Build history of the part. All positions in model axes, mm. Round coordinates to 2 decimals unless told otherwise and drop trailing zeros. Order: outer loops, then holes, each group sorted by start corner. A loop starts at its lowest first (then second) coordinate and runs counter-clockwise, first axis right, second up. Notation, with made-up numbers: (73.5, 15) - (128.5, 15) arc R29 cw to (128.5, 39) - close; hole circle Ø4 at (12.25, -18). An arc over 180 degrees is marked (long way). One line per question, with ' | ' between items. Start each with the question number.
from build123d import *

# Parameters (mm, degrees)
EXTRUDE_1_DEPTH   = 2
HOLE_WIZARD_M81_D = 9
CHAMFER_1_SIZE    = 2


with BuildPart() as part:
    # Эскиз1 → Бобышка-Вытянуть1 (new body)
    with BuildSketch(Plane(origin=(0, 0, 0), x_dir=(1, 0, 0), z_dir=(0, 0, -1))):
        Polygon((-75, 150), (75, 150), (75, 100), (25, 100), (25, 0), (-25, 0), (-25, 100), (-75, 100), align=None)
    extrude(amount=EXTRUDE_1_DEPTH)

    # Отверстие с зазором M81 (through all)
    with Locations(Plane(origin=(0, 0, -2), x_dir=(1, 0, 0), z_dir=(0, 0, -1))):
        with Locations((0, 25), (0, 125), (-50, 125), (50, 125), (0, 75)):
            Hole(HOLE_WIZARD_M81_D / 2)

    # Фаска1
    chamfer_1_edges = [part.edges().sort_by_distance(p)[0] for p in [
        (-75, -100, -1),
        (-75, -150, -1),
        (75, -150, -1),
        (75, -100, -1),
        (25, 0, -1),
        (-25, 0, -1),
    ]]
    chamfer(chamfer_1_edges, length=CHAMFER_1_SIZE)


solid = part.part
Item 1: Slice it at B-B (z = -0.4). Write the cut outline in (x, y), plus the area to 3 significant figures.
Item 2: Slice it at A-A (x = -50). Write the cut outline in (y, z).
Item 3: Wall check: line 1 along X through (y, z) = (-125, -0.55); line 2 along Y through (x, z) = (0, -1.1); line 3 along Y through (x, z) = (50, -1). Give the ranges that are in metal, low to high. Write a range as [from, to].
Item 4: Pin check, flat tips, straight feed: pin 1 (7 mm diameter, centred on x = 0, y = -125, fed in from -Z); pin 2 (1 mm diameter, centred on x = 39, z = -1, fed in from +Y); pin 3 (1 mm diameter, centred on y = -56.5, z = -1, fed in from -X); pin 4 (0.6 mm diameter, centred on y = -46.5, z = -1, fed in from +X). Stop position of each tip, or through.
Item 5: Slice it at D-D (x = 0). Write the cut outline in (y, z).
Item 6: Slice it at C-C (y = -25). Write the cut outline in (x, z), plus the area to 3 significant figures.
A:
1) outline: (-75, -148) - (-73, -150) - (73, -150) - (75, -148) - (75, -102) - (73, -100) - (25, -100) - (25, -2) - (23, 0) - (-23, 0) - (-25, -2) - (-25, -100) - (-73, -100) - (-75, -102) - close; hole circle Ø9 at (-50, -125); hole circle Ø9 at (0, -125); hole circle Ø9 at (0, -75); hole circle Ø9 at (0, -25); hole circle Ø9 at (50, -125) | area: 12,200 mm^2
2) outline: (-150, -2) - (-129.5, -2) - (-129.5, 0) - (-150, 0) - close; (-120.5, -2) - (-100, -2) - (-100, 0) - (-120.5, 0) - close
3) line 1: [-75, -54.5], [-45.5, -4.5], [4.5, 45.5], [54.5, 75] | line 2: [-150, -129.5], [-120.5, -79.5], [-70.5, -29.5], [-20.5, 0] | line 3: [-150, -129.5], [-120.5, -100]
4) pin 1: through | pin 2: y = -100 | pin 3: x = -25 | pin 4: x = 25
5) outline: (-150, -2) - (-129.5, -2) - (-129.5, 0) - (-150, 0) - close; (-120.5, -2) - (-79.5, -2) - (-79.5, 0) - (-120.5, 0) - close; (-70.5, -2) - (-29.5, -2) - (-29.5, 0) - (-70.5, 0) - close; (-20.5, -2) - (0, -2) - (0, 0) - (-20.5, 0) - close
6) outline: (-25, -2) - (-4.5, -2) - (-4.5, 0) - (-25, 0) - close; (4.5, -2) - (25, -2) - (25, 0) - (4.5, 0) - close | area: 82.0 mm^2
